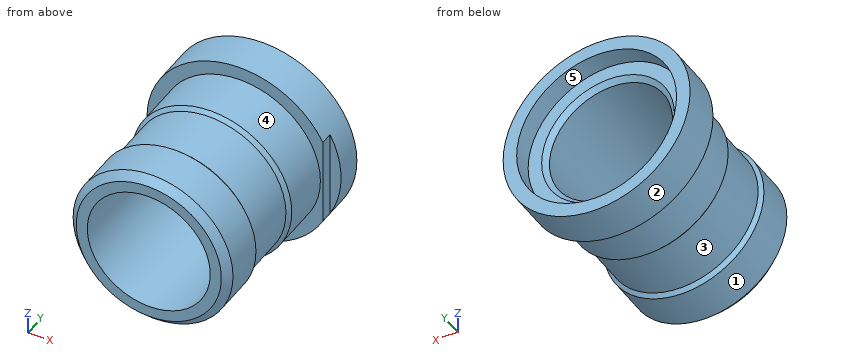
```python
from build123d import *

# Parameters (mm, degrees)
CUT_EXTRUDE1_START = -11
SKETCH2_W          = 20.025201173
SKETCH2_H          = 73.268677232
CUT_EXTRUDE1_DEPTH = 86.374270425
CHAMFER1_SIZE      = 3


with BuildPart() as part:
    # Sketch1 → Revolve1 (revolve)
    with BuildSketch(Plane.XY, mode=Mode.PRIVATE) as revolve1_sk:
        Polygon((-32.5, 80), (-32.5, 72), (-27, 72), (-25, 70), (-25, 0), (-32.5, 0), (-32.5, 19), (-31, 20.5), (-31, 42.5), (-32.5, 44), (-32.5, 64), (-38, 64), (-38, 80), align=None)
    revolve(revolve1_sk.sketch.rotate(Axis((0, 0, 0), (0, 1, 0)), 270), axis=Axis((0, 0, 0), (0, 1, 0)))

    # Sketch2 → Cut-Extrude1 (cut, through all)
    with BuildSketch(Plane(origin=(0, 80, 0), x_dir=(1, 0, 0), z_dir=(0, 1, 0)).offset(CUT_EXTRUDE1_START)):
        with Locations((43.512600586, -0.824567107)):
            Rectangle(SKETCH2_W, SKETCH2_H)
    extrude(amount=-CUT_EXTRUDE1_DEPTH, mode=Mode.SUBTRACT)

    # Chamfer1
    chamfer1_edges = [part.edges().sort_by_distance(p)[0] for p in [
        (0, 0, 32.5),
    ]]
    chamfer(chamfer1_edges, length=CHAMFER1_SIZE)


solid = part.part
```
The model under review builds one solid part; all positions refer to its coordinate system, in mm. Face numbers are marked on the shaded views. A direction names the side the tool comes from. Round coordinates to 2 decimals unless told otherwise and drop trailing zeros. Loops run counter-clockwise (first coordinate to the right, second up) from the corner with the lowest first, then second, coordinate; pieces in that order, holes last. Notation, with made-up numbers: (63, -38.5) -> (67, -38.5) arc R19 ccw to (67, -17.5) -> close; hole circle Ø11 at (27.5, -33.5). An arc over 180 degrees is marked (long way). Answer as a JSON object with one key per item and string values. Group by question number.
1) We need section A-A on x = 0. Write out the cut boundary in (y, z), then the cut area to 3 significant figures.
2) For line 1 (X direction, y = 5, z = -1); line 2 (X direction, y = 38, z = -0.5) (3 decimals); line 3 (Y direction, x = 16, z = 32), list the stretches that pass through material, from the lowest coordinate up. Write a range as [from, to].
3) For the marked faces 1, 2 and 3, list the 3-axis set-ups (+Z, -Z, +X, -X, +Y, -Y) from which the entire face can be reached by the end or side of a thin tool; tool diameter is ignored.
4) We need section C-C on y = 50.5. Write out the cut boundary in (x, z).
5) Mouldability with a two-part tool opening along Z and no side actions: class the marked faces 4 and 5 as released by +Z, released by -Z, zero draft, split by the parting line, or undercut.
6) For pin 1 Ø2.5 at (y, z) = (67, 5) entering from +X; pin 2 Ø1.4 at (x, z) = (35, -4) entering from -Y; pin 3 Ø8 at (y, z) = (54.5, 2) entering from +X, all flat-tipped, find the tip position at first contact; note any pin that passes through.
Result set:
{
 "1": {"outline": "(0, -29.5) -> (3, -32.5) -> (19, -32.5) -> (20.5, -31) -> (42.5, -31) -> (44, -32.5) -> (64, -32.5) -> (64, -38) -> (80, -38) -> (80, -32.5) -> (72, -32.5) -> (72, -27) -> (70, -25) -> (0, -25) -> close; (0, 25) -> (70, 25) -> (72, 27) -> (72, 32.5) -> (80, 32.5) -> (80, 38) -> (64, 38) -> (64, 32.5) -> (44, 32.5) -> (42.5, 31) -> (20.5, 31) -> (19, 32.5) -> (3, 32.5) -> (0, 29.5) -> close", "area": "1,170 mm²"},
 "2": {"line 1": "[-32.48, -24.98], [24.98, 32.48]", "line 2": "[-30.996, -24.995], [24.995, 30.996]", "line 3": "[64, 80]"},
 "3": {"face 1": "-Y", "face 2": "+Y, -Y", "face 3": "none"},
 "4": {"outline": "circle Ø65 at (0, 0); hole circle Ø50 at (0, 0)"},
 "5": {"face 4": "split by the parting line", "face 5": "undercut"},
 "6": {"pin 1": "x = 33.5", "pin 2": "y = 69", "pin 3": "x = 32.5"}
}
